Input: dimensioned drawing with shaded views. Units: mm. Origin: part minimum x, y, z. Round coordinates to 2 decimals unless told otherwise and drop trailing zeros. Order: outer loops, then holes, each group sorted by start corner. A loop starts at its lowest first (then second) coordinate and runs counter-clockwise, first axis right, second up. Notation, with made-up numbers: M -22,69 L 3,69 A26 cw 3,104 Z; hole C 75,81.25 d9. An arc over 180 degrees is marked long. Put each result on its own line as item: value. Start each with the question number.
1) Section A-A, the plane y = 10. Count the separate pieces of the cut face and the enclosed holes in it, then the cut area to 3 significant figures.
2) First-contact query: P1, Ø8, axis at x = 300, z = 100, coming from the -Y side; P2, Ø6, axis at y = 8.5, z = 138, coming from the -X side; P3, Ø4.5, axis at y = 7.5, z = 325.5, coming from the +X side. Flat tips, straight axial feed; report the tip coordinate or a pass-through.
3) Material intervals for probe 1 along Z at (x, y) = (300, 11.5); probe 2 along X at (y, z) = (11.5, 147), sorted ascending. Write a range as [from, to].
4) Section B-B, the plane z = 138. Return loops of the section in (x, y).
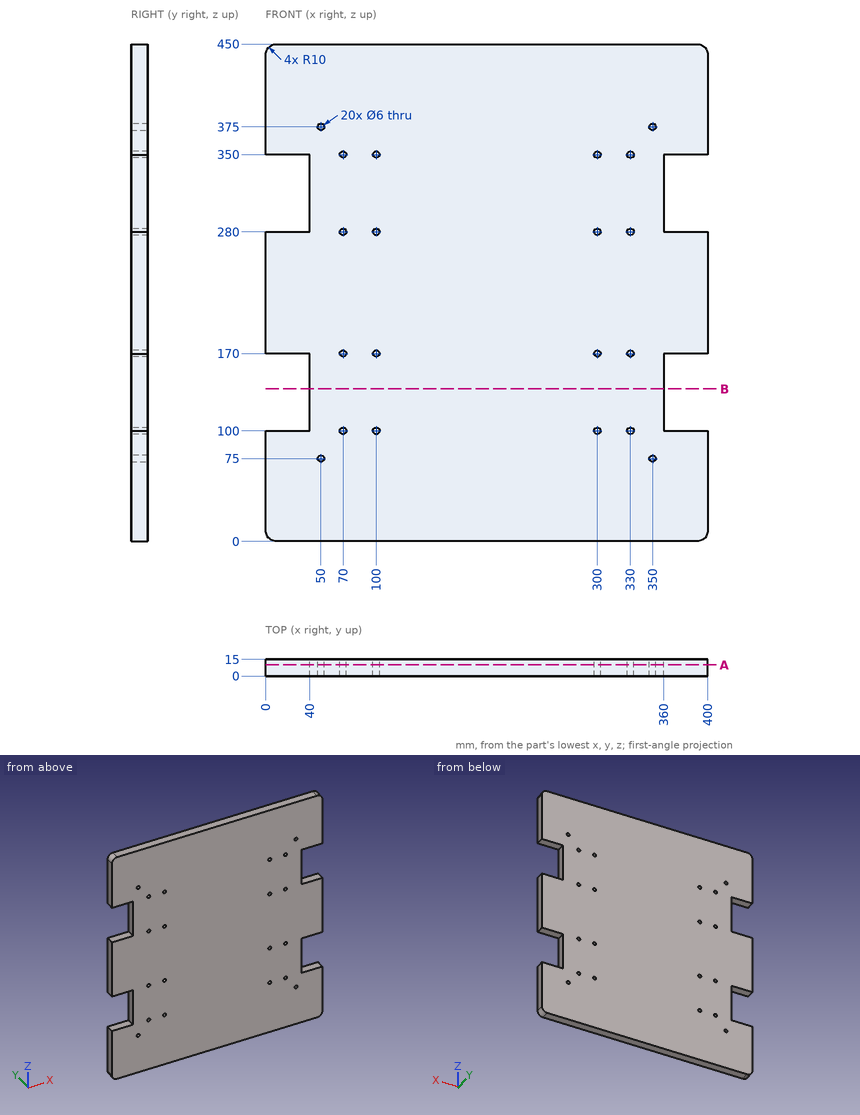
Result sheet:
1. separate pieces: 1
1. enclosed holes: 20
1. area: 168,000 mm2
2. P1: stops at y = 0
2. P2: stops at x = 40
2. P3: stops at x = 360
3. probe 1: z = [0, 97], [103, 167], [173, 277], [283, 347], [353, 450]
3. probe 2: x = [40, 360]
4. outline: M 40,0 L 360,0 L 360,15 L 40,15 Z
